Geometry: final body of the model. Coordinates: model frame, mm. Coordinates: 2 decimals unless noted, no trailing zeros. Loops run counter-clockwise (first coordinate to the right, second up) from the corner with the lowest first, then second, coordinate; pieces in that order, holes last. Notation, with made-up numbers: (26, 8) - (72, 8) arc R23 ccw to (72, 29) - close; hole circle Ø5 at (71, 71). An arc over 180 degrees is marked (long way). Answer in a Markdown table with one row per item.
from build123d import *

# Parameters (mm, degrees)
F1_DEPTH = 25.4


with BuildPart() as f1:
    # F0 (on Right) → F1 (new body)
    with BuildSketch(Plane.YZ):
        Polygon((127.646804, -74.149996), (0, 0), (-76.320149, 0), align=None)
        Polygon((96.973807, -116.791584), (127.646804, -74.149996), (-76.320149, 0), (82.375811, -141.921558), align=None)
    extrude(amount=F1_DEPTH)


solid = f1.part
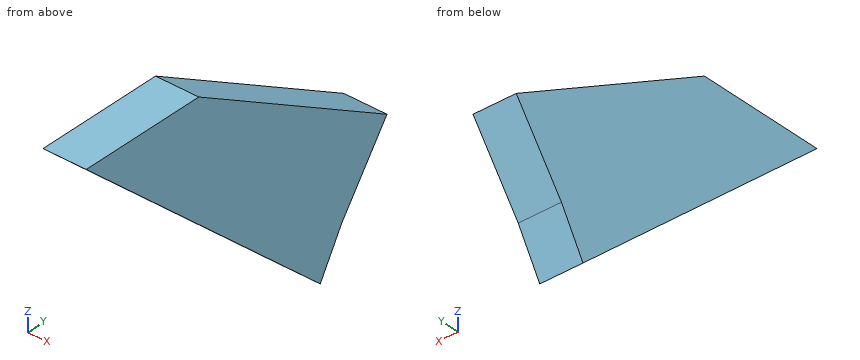
(1) Cut plane C-C on y = 67. Output: boundary loops of the cut face in (x, z).
Verdict:
| item | result |
|---|---|
| outline | (0, -128.17) - (25.4, -128.17) - (25.4, -38.92) - (0, -38.92) - close |
(2) First-contact query: pin 1 Ø5 at (x, z) = (15.5, -18) entering from -Y; pin 2 Ø4 at (x, z) = (15.5, -46) entering from -Y; pin 3 Ø1 at (x, y) = (4.5, -50) entering from -Z. Flat tips, straight axial feed; report the tip coordinate or a pass-through.
Verdict:
| item | result |
|---|---|
| pin 1 | stops at y = -58.99 |
| pin 2 | stops at y = -27.12 |
| pin 3 | stops at z = -23.99 |
(3) Ray query, probe 1 along Z at (x, y) = (2.5, 6); probe 2 along Z at (x, y) = (18.75, 0); probe 3 along Y at (x, z) = (11, -51.5). Return the intervals inside material, ascending.
Verdict:
| item | result |
|---|---|
| probe 1 | z = -73.62 to -3.49 |
| probe 2 | z = -68.25 to 0 |
| probe 3 | y = -18.73 to 88.66 |
(4) Cut plane A-A on x = 21. Output: boundary loops of the cut face in (y, z), then the cut area to 3 significant figures.
Verdict:
| item | result |
|---|---|
| outline | (-76.32, 0) - (82.38, -141.92) - (96.97, -116.79) - (127.65, -74.15) - (0, 0) - close |
| area | 11,300 mm² |
(5) Cut plane B-B on z = -112. Output: boundary loops of the cut face in (x, y), then the cut area to 3 significant figures.
Verdict:
| item | result |
|---|---|
| outline | (0, 48.92) - (25.4, 48.92) - (25.4, 100.42) - (0, 100.42) - close |
| area | 1,310 mm² |
